For this review, take the finished solid that the model builds, in its own axes (mm). Give positions to 0.01 mm unless a question says otherwise; leave off trailing zeros. Write each loop counter-clockwise with the first axis right and the second up, starting at its lowest first coordinate (ties: lowest second). Pieces come first, ordered by that corner, then holes.
1) Draft analysis for pull direction X (two halves, no side actions). For faces 1 (the face through (15, 0, 1)), 2 (the face through (5.69, 7.17, 1.01)), 3 (the face through (3, 3, 0)), state which applies: pulls with the +X half, pulls with the -X half, needs draft (parallel to the pull), parting line crosses it, or undercut.
2) We need section D-D on x = -3.5. Give the boundary of the cut face in (y, z), and give its area (3 significant figures).
3) Wall thickness on line 1 along Y through (x, z) = (-12, 1.05); line 2 along Y through (x, z) = (6, 0.8); line 3 along X through (y, z) = (-8, 1.25): over which ranges is each line inside the solid? List them lowest first.
4) We need section B-B on y = -6. Give the boundary of the cut face in (x, z), and give its area (3 significant figures).
5) We need section C-C on y = 8.5. Give the boundary of the cut face in (x, z), and give its area (3 significant figures).
6) We need section A-A on x = 5. Give the boundary of the cut face in (y, z).
from build123d import *

# Parameters (mm, degrees)
ESBO_O1_W                = 30
ESBO_O1_H                = 23
RESSALTO_EXTRUS_O1_DEPTH = 2
ESBO_O2_R                = 6.5
ESBO_O2_R_2              = 1.5
CORTE_EXTRUS_O1_DEPTH    = 20.006577809


with BuildPart() as part:
    # Esboço1 → Ressalto-extrusão1 (new body)
    with BuildSketch(Plane.XY):
        Rectangle(ESBO_O1_W, ESBO_O1_H)
    extrude(amount=RESSALTO_EXTRUS_O1_DEPTH)

    # Esboço2 → Corte-extrusão1 (cut, through all)
    with BuildSketch(Plane.XY.offset(2)):
        with Locations((-3.5, 0)):
            Circle(ESBO_O2_R)
        with Locations((5, 8.5)):
            Circle(ESBO_O2_R_2)
        with Locations(Location((5, -8.5, 0), (0, 0, 180))):
            Circle(ESBO_O2_R_2)
        with Locations((-12, -8.5)):
            Circle(ESBO_O2_R_2)
        with Locations(Location((-12, 8.5, 0), (0, 0, 180))):
            Circle(ESBO_O2_R_2)
    extrude(amount=-CORTE_EXTRUS_O1_DEPTH, mode=Mode.SUBTRACT)


solid = part.part
Results list:
1. face 1: pulls with the +X half
1. face 2: undercut
1. face 3: needs draft
2. outline: (-11.5, 0) - (-6.5, 0) - (-6.5, 2) - (-11.5, 2) - close; (6.5, 0) - (11.5, 0) - (11.5, 2) - (6.5, 2) - close
2. area: 20.0 mm2
3. line 1: y = -11.5 to -10, -7 to 7, 10 to 11.5
3. line 2: y = -11.5 to -9.62, -7.38 to 7.38, 9.62 to 11.5
3. line 3: x = -15 to -13.41, -10.59 to 3.59, 6.41 to 15
4. outline: (-15, 0) - (-6, 0) - (-6, 2) - (-15, 2) - close; (-1, 0) - (15, 0) - (15, 2) - (-1, 2) - close
4. area: 50.0 mm2
5. outline: (-15, 0) - (-13.5, 0) - (-13.5, 2) - (-15, 2) - close; (-10.5, 0) - (3.5, 0) - (3.5, 2) - (-10.5, 2) - close; (6.5, 0) - (15, 0) - (15, 2) - (6.5, 2) - close
5. area: 48.0 mm2
6. outline: (-11.5, 0) - (-10, 0) - (-10, 2) - (-11.5, 2) - close; (-7, 0) - (7, 0) - (7, 2) - (-7, 2) - close; (10, 0) - (11.5, 0) - (11.5, 2) - (10, 2) - close
